from build123d import *

# Parameters (mm, degrees)
SKETCH1_R               = 4.7625
BOSS_EXTRUDE1_DEPTH     = 2.778125
SKETCH5_OUTSIDE_W       = 66.676
SKETCH5_OUTSIDE_H       = 68.886
SKETCH5_OUTSIDE_R       = 7.14375
CUT_EXTRUDE2_DEPTH      = 13.245378593
CUT_EXTRUDE2_DRAFT      = -60
MIRROR1_COPY_1_SKETCH_W = 66.676
MIRROR1_COPY_1_SKETCH_H = 68.886
MIRROR1_COPY_1_SKETCH_R = 7.14375
MIRROR1_COPY_1_DEPTH    = 13.245378593
MIRROR1_COPY_1_DRAFT    = -60


with BuildPart() as part:
    # Sketch1 → Boss-Extrude1 (new, symmetric)
    with BuildSketch(Plane(origin=(0, 0, 0), x_dir=(1, 0, 0), z_dir=(0, 1, 0))):
        Polygon((-7.14375, 4.124445986), (-7.14375, -4.124445986), (0, -8.248891971), (7.14375, -4.124445986), (7.14375, 4.124445986), (0, 8.248891971), align=None)
        with Locations(Location((0, 0, 0), (0, 0, 270))):
            Circle(SKETCH1_R, mode=Mode.SUBTRACT)
    extrude(amount=BOSS_EXTRUDE1_DEPTH, both=True)


with BuildPart() as cut_extrude2_tool:
    # Sketch5 outside → Cut-Extrude2 (with draft: the straight prism first)
    with BuildSketch(Plane(origin=(0, 2.778125, 0), x_dir=(1, 0, 0), z_dir=(0, 1, 0))):
        Rectangle(SKETCH5_OUTSIDE_W, SKETCH5_OUTSIDE_H)
        Circle(SKETCH5_OUTSIDE_R, mode=Mode.SUBTRACT)
    extrude(amount=-CUT_EXTRUDE2_DEPTH)
    # Cut-Extrude2: the draft: its side faces are tilted about the plane it starts from
    cut_extrude2_sides = [cut_extrude2_tool.faces().sort_by_distance(p)[0] for p in [
        (0, -3.844564296, 34.443),
        (33.338, -3.844564296, 0),
        (0, -3.844564296, -34.443),
        (-33.338, -3.844564296, 0),
        (-7.14375, -3.844564296, 0),
    ]]
    draft(cut_extrude2_sides, Plane(origin=(0, 2.778125, 0), x_dir=(1, 0, 0), z_dir=(0, 1, 0)), CUT_EXTRUDE2_DRAFT)


with BuildPart() as part_1:
    add(part.part)

    # Cut-Extrude2: cut by cut_extrude2_tool
    add(cut_extrude2_tool.part, mode=Mode.SUBTRACT)


with BuildPart() as mirror1_copy_1_tool:
    # Mirror1 copy 1 sketch → Mirror1 copy 1 (with draft: the straight prism first)
    with BuildSketch(Plane.XZ.offset(2.778125)):
        Rectangle(MIRROR1_COPY_1_SKETCH_W, MIRROR1_COPY_1_SKETCH_H)
        Circle(MIRROR1_COPY_1_SKETCH_R, mode=Mode.SUBTRACT)
    extrude(amount=-MIRROR1_COPY_1_DEPTH)
    # Mirror1 copy 1: the draft: its side faces are tilted about the plane it starts from
    mirror1_copy_1_sides = [mirror1_copy_1_tool.faces().sort_by_distance(p)[0] for p in [
        (0, 3.844564296, 34.443),
        (33.338, 3.844564296, 0),
        (0, 3.844564296, -34.443),
        (-33.338, 3.844564296, 0),
        (-7.14375, 3.844564296, 0),
    ]]
    draft(mirror1_copy_1_sides, Plane.XZ.offset(2.778125), MIRROR1_COPY_1_DRAFT)


with BuildPart() as part_2:
    add(part_1.part)

    # Mirror1 copy 1: cut by mirror1_copy_1_tool
    add(mirror1_copy_1_tool.part, mode=Mode.SUBTRACT)


solid = part_2.part
Part model, mm, in its own coordinate system. Give positions to 0.01 mm unless a question says otherwise; leave off trailing zeros. Loops run counter-clockwise (first coordinate to the right, second up) from the corner with the lowest first, then second, coordinate; pieces in that order, holes last. Notation, with made-up numbers: M -3,23 L 39,23 A26 ccw 39,46 Z; hole C 69.5,37.25 d5. An arc over 180 degrees is marked long. Put each result on its own line as item: value. Start each with the question number.
1) Flat gauge pin, fed straight in: pin 1 (1 mm diameter, centred on x = -5.5, y = 1.5, fed in from +Z). Where does the tip first touch, or does it go through?
2) Probe probe 1 along X at (y, z) = (-0.9, 0); probe 2 along Z at (x, y) = (-4.25, 0.5); probe 3 along X at (y, z) = (1.4, -1.25). List the from-to ranges inside material, lowest first.
3) Pull direction X, two halves, no side cores. Call faces 1 (the conical face through (-6.406, 2.626, -3.719)), 2 (the cylindrical face through (-2.9, -0.04, -3.78)), 3 (the conical face through (6.424, -2.626, 3.688)): +X half, -X half, draft (parallel to the pull), parting line (faces both ways), or undercut.
4) Saw through at A-A (y = 0.25). List the corners of the cut face in (x, z) (1 decimal).
Numbers:
1. pin 1: z = 5.36
2. probe 1: -7.14 to -4.76, 4.76 to 7.14
2. probe 2: -5.8 to -2.15, 2.15 to 5.8
2. probe 3: -7.14 to -4.6, 4.6 to 7.14
3. face 1: -X half
3. face 2: undercut
3. face 3: +X half
4. outline: M -7.1,-4.1 L 0,-8.2 L 7.1,-4.1 L 7.1,4.1 L 0,8.2 L -7.1,4.1 Z; hole C 0,0 d9.5
